Could you check a few things on this drawing? It's one solid part, dimensions in mm from its lowest x, y, z. A direction names the side the tool comes from. Round coordinates to 2 decimals unless told otherwise and drop trailing zeros. Write each loop counter-clockwise with the first axis right and the second up, starting at its lowest first coordinate (ties: lowest second). Pieces come first, ordered by that corner, then holes. Notation, with made-up numbers: (47, 85.25) -> (65, 85.25) arc R25 cw to (65, 112.25) -> close; hole circle Ø6 at (54, -29). An arc over 180 degrees is marked (long way). Put each result on its own line as item: value. Start each with the question number.
1) I want a section at A-A, the plane z = 11.1. List the corners of the cut face in (x, y) for me.
2) I want a section at D-D, the plane z = 19.2. List the corners of the cut face in (x, y) for me, then the cut area to 3 significant figures.
3) Will these pins go through, and if not, where does the flat tip stop? P1, Ø5, axis at y = 2, z = 10.5, coming from the +X side; P2, Ø4.5, axis at x = 11.1, z = 19.2, coming from the +Y side; P3, Ø3, axis at x = 8, y = 12.5, coming from the +Z side.
4) I want a section at B-B, the plane x = 11.1. List the corners of the cut face in (y, z) for me, then the cut area to 3 significant figures.
5) We'd pull the mould along Z, two halves only. Please class the marked faces 1, 2 and 3: released by +Z, released by -Z, zero draft, split by the parting line, or undercut.
6) I want a section at C-C, the plane y = 11.75. List the corners of the cut face in (x, z) for me, then the cut area to 3 significant figures.
7) If I drill on line 1 along X through (y, z) = (12.4, 11.1); line 2 along X through (y, z) = (11.75, 12); line 3 along Y through (x, z) = (6.25, 8.5), over which ranges is the centre line in solid material (lowest first)? Write a range as [from, to].
8) Which directions (+Z, -Z, +X, -X, +Y, -Y) give clear straight access to the entire face, cutting with the end or side of a thin tool? Please do the marked faces 4 and 5.
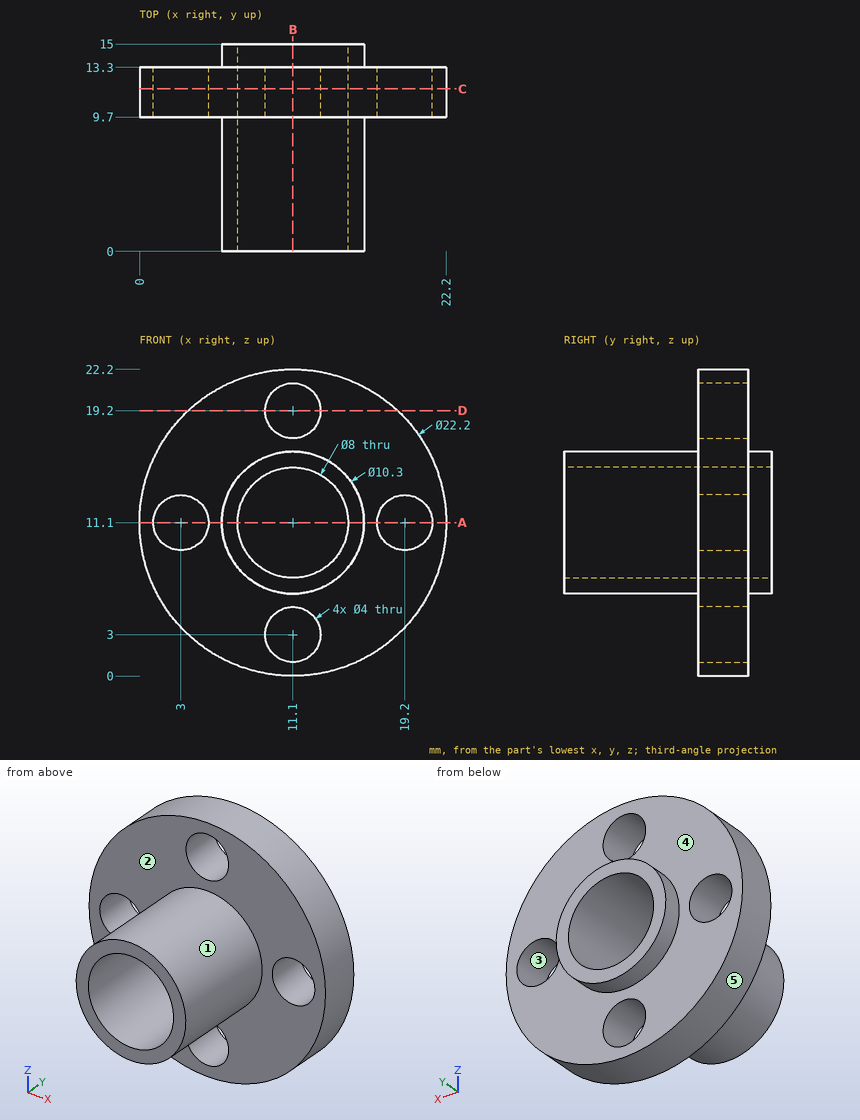
Findings:
1. outline: (0, 9.7) -> (1, 9.7) -> (1, 13.3) -> (0, 13.3) -> close; (5, 9.7) -> (5.95, 9.7) -> (5.95, 0) -> (7.1, 0) -> (7.1, 15) -> (5.95, 15) -> (5.95, 13.3) -> (5, 13.3) -> close; (15.1, 0) -> (16.25, 0) -> (16.25, 9.7) -> (17.2, 9.7) -> (17.2, 13.3) -> (16.25, 13.3) -> (16.25, 15) -> (15.1, 15) -> close; (21.2, 9.7) -> (22.2, 9.7) -> (22.2, 13.3) -> (21.2, 13.3) -> close
2. outline: (3.51, 9.7) -> (9.1, 9.7) -> (9.1, 13.3) -> (3.51, 13.3) -> close; (13.1, 9.7) -> (18.69, 9.7) -> (18.69, 13.3) -> (13.1, 13.3) -> close
2. area: 40.2 mm2
3. P1: stops at x = 16.25
3. P2: stops at y = 13.3
3. P3: stops at z = 22.08
4. outline: (0, 5.95) -> (9.7, 5.95) -> (9.7, 5) -> (13.3, 5) -> (13.3, 5.95) -> (15, 5.95) -> (15, 7.1) -> (0, 7.1) -> close; (0, 15.1) -> (15, 15.1) -> (15, 16.25) -> (13.3, 16.25) -> (13.3, 17.2) -> (9.7, 17.2) -> (9.7, 16.25) -> (0, 16.25) -> close; (9.7, 0) -> (13.3, 0) -> (13.3, 1) -> (9.7, 1) -> close; (9.7, 21.2) -> (13.3, 21.2) -> (13.3, 22.2) -> (9.7, 22.2) -> close
4. area: 48.5 mm2
5. face 1: split by the parting line
5. face 2: zero draft
5. face 3: undercut
6. outline: circle Ø22.2 at (11.1, 11.1); hole circle Ø4 at (3, 11.1); hole circle Ø8 at (11.1, 11.1); hole circle Ø4 at (11.1, 3); hole circle Ø4 at (11.1, 19.2); hole circle Ø4 at (19.2, 11.1)
6. area: 287 mm2
7. line 1: x = [0, 1], [5, 7.1], [15.1, 17.2], [21.2, 22.2]
7. line 2: x = [0.04, 1.21], [4.79, 7.2], [15, 17.41], [20.99, 22.16]
7. line 3: y = [9.7, 13.3]
8. face 4: +Y
8. face 5: +Y, -Y
